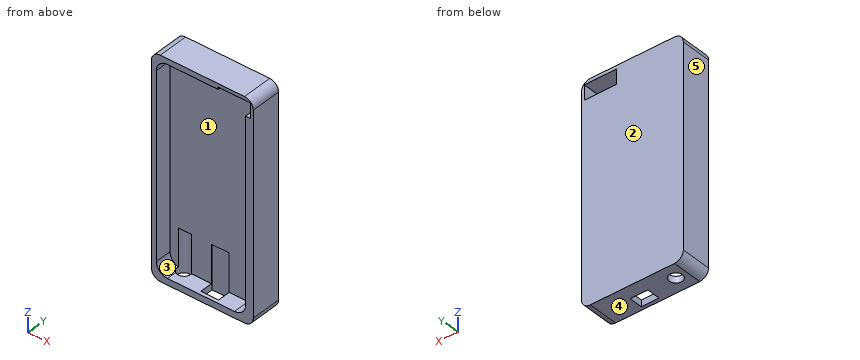
from build123d import *

# Parameters (mm, degrees)
F0_W     = 58.42
F0_H     = 124.46
F1_DEPTH = 17.526
F3_DEPTH = 9.398
F6_R     = 5.08
F4_W     = 18.451236
F4_H     = 8.469313
F7_DEPTH = 25.4
F5_R     = 3.81
F5_W     = 10.16
F5_H     = 7.80597
F8_DEPTH = 25.4


with BuildPart() as f1:
    # F0 (on Front) → F1 (new body)
    with BuildSketch(Plane.XZ):
        with Locations((29.21, 62.23)):
            Rectangle(F0_W, F0_H)
    extrude(amount=F1_DEPTH)

    # F2 (on face) → F3 (cut)
    with BuildSketch(Plane.XZ.offset(17.526)):
        with BuildLine():
            ThreePointArc((2.862678, 10.059572), (4.72255, 5.569444), (9.212678, 3.709572))
            Line((9.212678, 3.709572), (47.659166, 3.709572))
            ThreePointArc((47.659166, 3.709572), (52.149294, 5.569444), (54.009166, 10.059572))
            Line((54.009166, 10.059572), (54.009166, 114.920157))
            ThreePointArc((54.009166, 114.920157), (52.149294, 119.410285), (47.659166, 121.270157))
            Line((47.659166, 121.270157), (9.212678, 121.270157))
            ThreePointArc((9.212678, 121.270157), (4.72255, 119.410285), (2.862678, 114.920157))
            Line((2.862678, 114.920157), (2.862678, 10.059572))
        make_face()
    extrude(amount=-F3_DEPTH, mode=Mode.SUBTRACT)

    # F6
    f6_edges = [f1.edges().sort_by_distance(p)[0] for p in [
        (0, -8.763, 124.46),
        (58.42, -8.763, 124.46),
        (58.42, -8.763, 0),
        (0, -8.763, 0),
    ]]
    fillet(f6_edges, radius=F6_R)

    # F4 (on Front) → F7 (cut)
    with BuildSketch(Plane.XZ):
        with Locations((47.542691, 118.296183)):
            Rectangle(F4_W, F4_H)
    extrude(amount=F7_DEPTH, mode=Mode.SUBTRACT)

    # F5 (on face) → F8 (cut)
    with BuildSketch(Plane(origin=(0, 0, 0), x_dir=(1, 0, 0), z_dir=(0, 0, -1))):
        with Locations((11.43, 8.70138)):
            Circle(F5_R)
        with Locations((31.753567, 11.591015)):
            Rectangle(F5_W, F5_H)
    extrude(amount=-F8_DEPTH, mode=Mode.SUBTRACT)


solid = f1.part
Read the model definition and answer for the solid it produces. Units are mm, in the model's axes. Face numbers are marked on the shaded views. A direction names the side the tool comes from. Round coordinates to 2 decimals unless told otherwise and drop trailing zeros. Loops run counter-clockwise (first coordinate to the right, second up) from the corner with the lowest first, then second, coordinate; pieces in that order, holes last.
Q1. Determine the mould class of the marked faces 3, 4 and 5 for opening direction X: released by +X, released by -X, zero draft, split by the parting line, or undercut.
Q2. Section D-D on z = 109 is taken. Write down the section's boundary in (x, y), and give its area (3 significant figures).
Q3. Section A-A on x = 11.43 is taken. Write down the section's boundary in (y, z).
Q4. Section C-C on x = 22.5 is taken. Write down the section's boundary in (y, z).
Q5. Each of these flat-tipped pins is pushed along its axis until it touches: pin 1 (1 mm diameter, centred on x = 13.5, y = -6.5, fed in from -Z); pin 2 (7.5 mm diameter, centred on x = 18, y = -12.5, fed in from -Z); pin 3 (8 mm diameter, centred on x = 33, z = 11, fed in from -Y). Where does it stop, or does it pass through?
Q6. Section B-B on y = -2 is taken. Write down the section's boundary in (x, z).
Q7. Which of the six approach directions +Z, -Z, +X, -X, +Y, -Y give full straight-line access (tool end or side, diameter ignored) to the marked faces 1 and 2?
Q8. Consider probe 1 along Z at (x, y) = (9.5, -14); probe 2 along X at (y, z) = (-13, 83); probe 3 along Z at (x, y) = (51, -8). Determine where each line is inside the solid, lowest interval first.
Output:
1. face 3: undercut
1. face 4: zero draft
1. face 5: released by -X
2. outline: (0, -17.53) - (2.86, -17.53) - (2.86, -8.13) - (54.01, -8.13) - (54.01, -17.53) - (58.42, -17.53) - (58.42, 0) - (0, 0) - close
2. area: 543 mm2
3. outline: (-17.53, 0) - (-12.51, 0) - (-12.51, 3.71) - (-17.53, 3.71) - close; (-17.53, 121.27) - (-8.13, 121.27) - (-8.13, 25.4) - (-4.89, 25.4) - (-4.89, 0) - (0, 0) - (0, 124.46) - (-17.53, 124.46) - close
4. outline: (-17.53, 0) - (0, 0) - (0, 124.46) - (-17.53, 124.46) - (-17.53, 121.27) - (-8.13, 121.27) - (-8.13, 3.71) - (-17.53, 3.71) - close
5. pin 1: stops at z = 25.4
5. pin 2: stops at z = 0
5. pin 3: stops at y = -8.13
6. outline: (0, 5.08) arc R5.08 ccw to (5.08, 0) - (53.34, 0) arc R5.08 ccw to (58.42, 5.08) - (58.42, 119.38) arc R5.08 ccw to (53.34, 124.46) - (5.08, 124.46) arc R5.08 ccw to (0, 119.38) - close; hole (38.32, 114.06) - (56.77, 114.06) - (56.77, 122.53) - (38.32, 122.53) - close
7. face 1: -Y
7. face 2: +Z, -Z, +X, -X, +Y
8. probe 1: z = 0 to 3.71, 121.27 to 124.46
8. probe 2: x = 0 to 2.86, 54.01 to 58.42
8. probe 3: z = 0 to 114.06, 122.53 to 124.46
